The listing builds one solid part. Answer for the finished solid, in the listing's coordinates (mm). A direction names the side the tool comes from. Give positions to 0.01 mm unless a question says otherwise; leave off trailing zeros. Write each loop counter-clockwise with the first axis right and the second up, starting at its lowest first coordinate (ties: lowest second). Pieces come first, ordered by that corner, then holes. Notation, with made-up numbers: (16, 2) - (30, 2) arc R20 ccw to (30, 22) - close; hole circle Ø7 at (-4, 63). An arc over 180 degrees is marked (long way). Use a Markdown table: item, result. Add a question column.
from build123d import *

# Parameters (mm, degrees)
CROQUIS1_R              = 2.7
SALIENTE_EXTRUIR1_DEPTH = 10
SALIENTE_EXTRUIR2_DEPTH = 10


with BuildPart() as part:
    # Croquis1 → Saliente-Extruir1 (new body, symmetric)
    with BuildSketch(Plane(origin=(0, 0, 0), x_dir=(1, 0, 0), z_dir=(0, 1, 0))):
        Circle(CROQUIS1_R)
    extrude(amount=SALIENTE_EXTRUIR1_DEPTH, both=True)

    # Croquis2 → Saliente-Extruir2 (add)
    with BuildSketch(Plane(origin=(0, 10, 0), x_dir=(1, 0, 0), z_dir=(0, 1, 0))):
        with BuildLine():
            Line((1.966596, 1.85), (-1.966596, 1.85))
            ThreePointArc((-1.966596, 1.85), (-2.7, 0), (-1.966596, -1.85))
            Line((-1.966596, -1.85), (1.966596, -1.85))
            ThreePointArc((1.966596, -1.85), (2.7, 0), (1.966596, 1.85))
        make_face()
    saliente_extruir2 = extrude(amount=SALIENTE_EXTRUIR2_DEPTH)

    # Simetría1: Saliente-Extruir2 across plane
    add(saliente_extruir2.mirror(Plane.ZX))


solid = part.part
1. Consider L1, parallel to Z at x = -1.7, y = 10.5; L2, parallel to Z at x = -0.15, y = -2; L3, parallel to Y at x = 1, z = -2.3. Determine where each line is inside the solid, lowest interval first. Write a range as [from, to].
2. The part is cut by section B-B (z = 1.15). Give the vertices of the cut face in (x, y), and give its area (3 significant figures).
3. The part is cut by section A-A (x = 0). Give the vertices of the cut face in (y, z).
4. The part is cut by section C-C (y = 15). Give the vertices of the cut face in (x, z).
5. Which of the six approach directions +Z, -Z, +X, -X, +Y, -Y give full straight-line access (tool end or side, diameter ignored) to faces 1 (the flat face through (0, 15, 1.85)), 2 (the flat face through (0, -10, 2.2)), 3 (the flat face through (0, 10, -2.2))?
6. Given P1, Ø1.2, axis at x = 0.5, y = 14, coming from the +Z side; P2, Ø3, axis at x = -1, y = -16, coming from the -Z side; P3, Ø0.7, axis at x = -1, z = 2.5, coming from the -Y side, each flat-ended and moving along its own axis, determine where each tip first touches the part or whether it passes through.
7. The part is cut by section D-D (y = -3.5). Give the vertices of the cut face in (x, z).
Check values:
| question | item | result |
|---|---|---|
| 1 | L1 | z = [-1.85, 1.85] |
| 1 | L2 | z = [-2.7, 2.7] |
| 1 | L3 | y = [-10, 10] |
| 2 | outline | (-2.44, -20) - (2.44, -20) - (2.44, 20) - (-2.44, 20) - close |
| 2 | area | 195 mm2 |
| 3 | outline | (-20, -1.85) - (-10, -1.85) - (-10, -2.7) - (10, -2.7) - (10, -1.85) - (20, -1.85) - (20, 1.85) - (10, 1.85) - (10, 2.7) - (-10, 2.7) - (-10, 1.85) - (-20, 1.85) - close |
| 4 | outline | (-1.97, -1.85) - (1.97, -1.85) arc R2.7 ccw to (1.97, 1.85) - (-1.97, 1.85) arc R2.7 ccw to start |
| 5 | face 1 | +Z, +X, -X, +Y |
| 5 | face 2 | +Z, +X, -X, -Y |
| 5 | face 3 | -Z, +X, -X, +Y |
| 6 | P1 | stops at z = 1.85 |
| 6 | P2 | stops at z = -1.85 |
| 6 | P3 | stops at y = -10 |
| 7 | outline | circle Ø5.4 at (0, 0) |
